Geometry: final body of the model. Coordinates: model frame, mm. Face numbers are marked on the shaded views. Coordinates: 2 decimals unless noted, no trailing zeros. Order: outer loops, then holes, each group sorted by start corner. A loop starts at its lowest first (then second) coordinate and runs counter-clockwise, first axis right, second up. Notation, with made-up numbers: (59.25, -39.5) -> (107.25, -39.5) arc R28 ccw to (107.25, -13.5) -> close; hole circle Ø6 at (-10.5, -8.5). An arc over 180 degrees is marked (long way). Answer in a Markdown table with one row per item. Add a question column.
1) Pull-direction query (X, two-part tool) for the marked faces 1 and 2; classes: +X half, -X half, draft (parallel to the pull), parting line (faces both ways), or undercut.
2) Section query C-C on x = -6. Return the cut outline in (y, z).
3) Section query B-B on z = 0. Return the cut outline in (x, y), then the cut area to 3 significant figures.
4) Ray query, line 1 (Y direction, x = 0, z = 9.2); line 2 (Z direction, x = 0, y = 53.5). Return the intervals inside material, ascending. Write a range as from..to.
5) Section query A-A on x = 0. Return the cut outline in (y, z), then the cut area to 3 significant figures.
6) Section query D-D on y = 116. Return the cut outline in (x, z).
7) Contact query for flat-ended pins moving along their axis: P1, Ø1, axis at x = -6.5, y = 75, coming from the +Z side; P2, Ø1, axis at y = 31, z = -0.5, coming from the +X side; P3, Ø2.5, axis at x = 0, y = 12.5, coming from the -Z side; P4, Ø6, axis at y = 142.5, z = 6.5, coming from the +X side. Output: stop coordinate, or through.
```python
from build123d import *

# Parameters (mm, degrees)
SKETCH1_R           = 10
SKETCH1_R_2         = 9
BOSS_EXTRUDE1_DEPTH = 162
SKETCH3_R           = 2
CUT_EXTRUDE2_DEPTH  = 21


with BuildPart() as part:
    # Sketch1 → Boss-Extrude1 (new body)
    with BuildSketch(Plane(origin=(0, 0, 0), x_dir=(1, 0, 0), z_dir=(0, 1, 0))):
        Circle(SKETCH1_R)
        Circle(SKETCH1_R_2, mode=Mode.SUBTRACT)
    extrude(amount=BOSS_EXTRUDE1_DEPTH)

    # Sketch3 → Cut-Extrude2 (cut, through all)
    with BuildSketch(Plane.XY.offset(10)):
        with Locations((0, 149.5)):
            Circle(SKETCH3_R)
        with Locations((0, 12.5)):
            Circle(SKETCH3_R)
    extrude(amount=-CUT_EXTRUDE2_DEPTH, mode=Mode.SUBTRACT)


solid = part.part
```
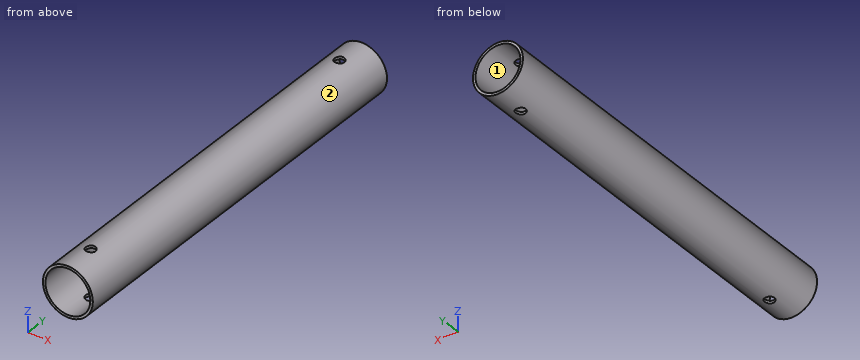
Result:
| question | item | result |
|---|---|---|
| 1 | face 1 | undercut |
| 1 | face 2 | parting line |
| 2 | outline | (0, -8) -> (162, -8) -> (162, -6.71) -> (0, -6.71) -> close; (0, 6.71) -> (162, 6.71) -> (162, 8) -> (0, 8) -> close |
| 3 | outline | (-10, 0) -> (-9, 0) -> (-9, 162) -> (-10, 162) -> close; (9, 0) -> (10, 0) -> (10, 162) -> (9, 162) -> close |
| 3 | area | 324 mm2 |
| 4 | line 1 | 0..10.5, 14.5..147.5, 151.5..162 |
| 4 | line 2 | -10..-9, 9..10 |
| 5 | outline | (0, -10) -> (10.5, -10) -> (10.5, -9) -> (0, -9) -> close; (0, 9) -> (10.5, 9) -> (10.5, 10) -> (0, 10) -> close; (14.5, -10) -> (147.5, -10) -> (147.5, -9) -> (14.5, -9) -> close; (14.5, 9) -> (147.5, 9) -> (147.5, 10) -> (14.5, 10) -> close; (151.5, -10) -> (162, -10) -> (162, -9) -> (151.5, -9) -> close; (151.5, 9) -> (162, 9) -> (162, 10) -> (151.5, 10) -> close |
| 5 | area | 308 mm2 |
| 6 | outline | circle Ø20 at (0, 0); hole circle Ø18 at (0, 0) |
| 7 | P1 | z = 8 |
| 7 | P2 | x = 10 |
| 7 | P3 | through |
| 7 | P4 | x = 9.37 |
